from build123d import *

# Parameters (mm, degrees)
F3_DEPTH = 1.27
F5_DEPTH = 20.32


# Not quite as in the source:
# - the dataset's text gives a spline's control points without its knots; the knots are read off the source's solid


with BuildPart() as f1:
    # F0 (on Right) → F1 (revolve)
    with BuildSketch(Plane.YZ):
        with BuildLine():
            Line((-5.5626, 0), (-3.175, 0))
            add(Edge.make_bspline(
                [(-3.175, 0), (-3.175, 10.541), (-4.0239762357, 25.9589322905), (-0.7943624519, 30.4792560231), (0, 31.75)],
                knots=[0, 0, 0, 0, 0.6813666235, 1, 1, 1, 1], degree=3))
            Line((0, 31.75), (0, 34.1376))
            ThreePointArc((0, 34.1376), (-1.1573462176, 33.8383446776), (-2.0245751497, 33.015594415))
            add(Edge.make_bspline(
                [(-5.5626, 0), (-5.5626, 1.9177725401), (-5.6012595175, 5.763256361), (-5.6850380944, 11.3740945743), (-5.7026900101, 16.6481342132), (-5.5838020802, 20.622627977), (-5.3557319657, 23.480741035), (-5.1437190397, 25.1246883423), (-4.9215103036, 26.3507670581), (-4.7229256392, 27.2307815663), (-4.4932831777, 28.052608441), (-4.1541081797, 29.0674517161), (-3.6792176979, 30.1931579589), (-2.8749355371, 31.7097687785), (-2.3121014901, 32.5556376731), (-2.0245751497, 33.015594415)],
                knots=[0, 0, 0, 0, 0.1249999999, 0.2499999998, 0.3749999996, 0.4999999995, 0.5624999995, 0.6249999994, 0.6562499994, 0.6874999993, 0.7187499993, 0.7499999993, 0.8124999992, 0.8749999991, 0.999999999, 0.999999999, 0.999999999, 0.999999999], degree=3))
        make_face()
    revolve(axis=Axis((0, -4.3688, 0), (0, 1, 0)))

    # F2 (on Front) → F3 (join)
    with BuildSketch(Plane.XZ):
        with BuildLine():
            Line((10.16, -34.2715069771), (10.16, -30.0805069771))
            ThreePointArc((10.16, -30.0805069771), (0, -31.75), (-10.16, -30.0805069771))
            Line((-10.16, -30.0805069771), (-10.16, -34.2715069771))
            Line((-10.16, -34.2715069771), (10.16, -34.2715069771))
        make_face()
    extrude(amount=F3_DEPTH)

    # F4 (on face) → F5 (join)
    with BuildSketch(Plane.YZ.offset(10.16)):
        Polygon((-0.635, -33.1716547143), (-1.27, -34.2715069771), (0.8637133898, -35.5034069771), (1.4987133898, -34.4035547143), align=None)
    extrude(amount=-F5_DEPTH)


solid = f1.part
Model file for the job. Use its own axes, mm. A direction names the side the tool comes from. Give positions to 0.01 mm unless a question says otherwise; leave off trailing zeros. Write item = value, one per line. Start each with the question number.
1. Drop flat-ended pins along their axis: P1, Ø3, axis at x = -12.5, z = 5.5, coming from the +Y side; P2, Ø4, axis at x = -8.5, y = -3.5, coming from the -Z side; P3, Ø12, axis at x = -3, z = 2, coming from the -Y side. Give the stop position or say it passes through.
2. Probe line 1 along Y through (x, z) = (16.5, 3); line 2 along X through (y, z) = (-0.75, 17.5); line 3 along Z through (x, y) = (3.5, -0.5). List the from-to ranges inside material, lowest first.
3. Which spindle directions (+Z, -Z, +X, -X, +Y, -Y) get a long thin tool onto all of the face, cutting with end or side? Do faces 1 (the flat face through (0, -1.27, -34)), 2 (the flat face through (20, 0, -25)), 3 (the flat face through (0.14, -0.22, -34.88)). Say none if no direction does.
Taken from the geometry:
q1.P1 = -3.29
q1.P2 = -32.59
q1.P3 = -5.66
q2.line_1 = -5.67 to -3.29
q2.line_2 = -29.17 to -25.04, 25.04 to 29.17
q2.line_3 = -34.72 to -30.76, 30.76 to 33.9
q3.face_1 = -Z, -Y
q3.face_2 = +Z, +X, -X, +Y
q3.face_3 = -Z, +X, -X, -Y
